Could you check a few things on this model? Use its own coordinates, in mm. Face numbers are marked on the shaded views. A direction names the side the tool comes from. Give positions to 0.01 mm unless a question says otherwise; leave off trailing zeros. Loops run counter-clockwise (first coordinate to the right, second up) from the corner with the lowest first, then second, coordinate; pieces in that order, holes last. Notation, with made-up numbers: (-24, -9.75) - (-15, -9.75) arc R27 ccw to (-15, 21.25) - close; hole circle Ø1 at (83, -8). An arc over 180 degrees is marked (long way). Write each question's results on one line, items separated by ' | '. Start each with the question number.
(1) On a 3-axis mill with a long thin cutter (end or side, diameter ignored), from which of +Z, -Z, +X, -X, +Y, -Y can I reach the whole of each face in a straight line? I mean the marked faces 1 and 2. Say none if no direction works.
(2) For pin 1 (12 mm diameter, centred on x = -17, z = 2.5, fed in from -Y); pin 2 (1 mm diameter, centred on x = 14, z = 11.5, fed in from +Y); pin 3 (3 mm diameter, centred on x = 28.5, z = 4.5, fed in from +Y), each with a flat end and sliding along its axis, tell me the tip position at first contact or that it passes through.
(3) Suppose I cut it at C-C (z = 9). Please give me the cut outline in (x, y), and give its area (3 significant figures).
(4) I need wall thicknesses on line 1 (Y direction, x = 0, z = 8.5); line 2 (Z direction, x = 28, y = -8); line 3 (Y direction, x = -24.5, z = 13.25). Which ranges of each line are inside material? Lowest first, please.
from build123d import *

# Parameters (mm, degrees)
F0_R     = 43
F1_DEPTH = 2
F0_R_2   = 45
F2_DEPTH = 25
F3_R     = 1.99999


# Not quite as in the source:
# - a fillet or chamfer is up to 0.001 mm smaller than in the source, because OpenCascade refuses the exact size


with BuildPart() as f1:
    # F0 (on Top) → F1 (new body)
    with BuildSketch(Plane.XY):
        Circle(F0_R)
    extrude(amount=F1_DEPTH)

    # F0 (on Top) → F2 (join)
    with BuildSketch(Plane.XY):
        Circle(F0_R_2)
        Circle(F0_R, mode=Mode.SUBTRACT)
    extrude(amount=F2_DEPTH)

    # F3 (radius 2 in the source; OpenCascade refuses exactly that, so slightly less here)
    f3_edges = [f1.edges().sort_by_distance(p)[0] for p in [
        (-45, 0, 0),
        (-45, 0, 25),
    ]]
    fillet(f3_edges, radius=F3_R)


solid = f1.part
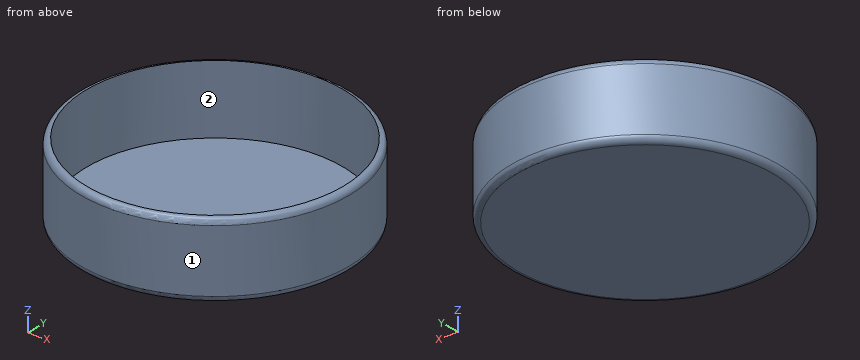
Output values:
1) face 1: +Z, -Z | face 2: +Z
2) pin 1: y = -43.63 | pin 2: y = 42.93 | pin 3: y = 36
3) outline: circle Ø90 at (0, 0); hole circle Ø86 at (0, 0) | area: 553 mm2
4) line 1: -45 to -43, 43 to 45 | line 2: 0 to 2 | line 3: -37.75 to -35.34, 35.34 to 37.75
